Can you work these out from the model? Positions are in its coordinate system, mm. Face numbers are marked on the shaded views. A direction names the side the tool comes from. Coordinates: 2 decimals unless noted, no trailing zeros. Write each loop counter-clockwise with the first axis right and the second up, starting at its lowest first coordinate (ties: lowest second). Pieces come first, ordered by that corner, then holes. Notation, with made-up numbers: (32.25, 33.25) -> (46.25, 33.25) arc R18 cw to (46.25, 46.25) -> close; hole circle Ø3 at (35, 18). An arc over 180 degrees is marked (long way). Use one line per item in the form item = value.
```python
from build123d import *

# Parameters (mm, degrees)
SKETCH1_W           = 60
SKETCH1_H           = 60
BOSS_EXTRUDE1_DEPTH = 6
SKETCH2_W           = 6
SKETCH2_H           = 16
SKETCH2_W_2         = 5.95
SKETCH2_H_2         = 15.95
SKETCH2_W_3         = 5.9
SKETCH2_H_3         = 15.9
SKETCH2_W_4         = 5.85
SKETCH2_H_4         = 15.85
SKETCH2_W_5         = 5.8
SKETCH2_H_5         = 15.8
SKETCH2_W_6         = 5.75
SKETCH2_H_6         = 15.75
CUT_EXTRUDE1_DEPTH  = 6
SKETCH3_W           = 15.128686335
SKETCH3_H           = 1.558081165
CUT_EXTRUDE2_DEPTH  = 6
SKETCH4_W           = 60
SKETCH4_H           = 14.757524832
CUT_EXTRUDE3_DEPTH  = 6


with BuildPart() as part:
    # Sketch1 → Boss-Extrude1 (new body)
    with BuildSketch(Plane(origin=(0, 0, 0), x_dir=(1, 0, 0), z_dir=(0, 1, 0))):
        with Locations((30, 30)):
            Rectangle(SKETCH1_W, SKETCH1_H)
    extrude(amount=BOSS_EXTRUDE1_DEPTH)

    # Sketch2 → Cut-Extrude1 (cut)
    with BuildSketch(Plane(origin=(0, 6, 0), x_dir=(1, 0, 0), z_dir=(0, 1, 0))):
        with Locations((6, 47)):
            Rectangle(SKETCH2_W, SKETCH2_H)
        with Locations((18, 47)):
            Rectangle(SKETCH2_W, SKETCH2_H)
        with Locations((30.15, 47)):
            Rectangle(SKETCH2_W, SKETCH2_H)
        with Locations((42.4, 47)):
            Rectangle(SKETCH2_W, SKETCH2_H)
        with Locations((54.75, 47)):
            Rectangle(SKETCH2_W, SKETCH2_H)
        with Locations((5.975, 25.682524832)):
            Rectangle(SKETCH2_W_2, SKETCH2_H_2)
        with Locations((17.95, 25.707524832)):
            Rectangle(SKETCH2_W_3, SKETCH2_H_3)
        with Locations((30.075, 25.732524832)):
            Rectangle(SKETCH2_W_4, SKETCH2_H_4)
        with Locations((42.3, 25.757524832)):
            Rectangle(SKETCH2_W_5, SKETCH2_H_5)
        with Locations((54.625, 25.782524832)):
            Rectangle(SKETCH2_W_6, SKETCH2_H_6)
    extrude(amount=-CUT_EXTRUDE1_DEPTH, mode=Mode.SUBTRACT)

    # Sketch3 → Cut-Extrude2 (cut)
    with BuildSketch(Plane(origin=(0, 6, 0), x_dir=(1, 0, 0), z_dir=(0, 1, 0))):
        with Locations((30.785905784, 59.220959418)):
            Rectangle(SKETCH3_W, SKETCH3_H)
    extrude(amount=-CUT_EXTRUDE2_DEPTH, mode=Mode.SUBTRACT)

    # Sketch4 → Cut-Extrude3 (cut)
    with BuildSketch(Plane(origin=(0, 6, 0), x_dir=(1, 0, 0), z_dir=(0, 1, 0))):
        with Locations((30, 7.378762416)):
            Rectangle(SKETCH4_W, SKETCH4_H)
    extrude(amount=-CUT_EXTRUDE3_DEPTH, mode=Mode.SUBTRACT)


solid = part.part
```
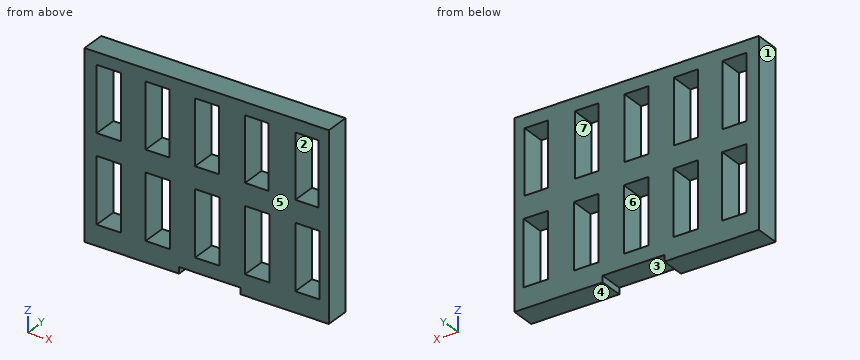
Q1. Suppose I cut it at D-D (y = 3.4). Give the number of separate pieces and of enclosed holes in the cut face, then the cut area to 3 significant figures.
Return value:
separate_pieces = 1
enclosed_holes = 10
area = 1,750 mm2
Q2. If I drill on line 1 (X direction, y = 3.75, z = -43.5); line 2 (Z direction, x = 56, y = 5.45); line 3 (X direction, y = 4, z = -18), over which ranges is the centre line in solid material (lowest first)? Write a range as from..to.
Return value:
line_1 = 0..3, 9..15, 21..27.15, 33.15..39.4, 45.4..51.75, 57.75..60
line_2 = -60..-55, -39..-33.66, -17.91..-14.76
line_3 = 0..3, 8.95..15, 20.9..27.15, 33..39.4, 45.2..51.75, 57.5..60
Q3. Thinking about a two-plate mould opening in Z: for the marked faces 4, 5, 6 and 7, which applies, released by +Z, released by -Z, zero draft, split by the parting line, or undercut?
Return value:
face_4 = released by -Z
face_5 = zero draft
face_6 = undercut
face_7 = undercut
Q4. Suppose I cut it at C-C (x = 8). Write out the boundary of the cut face in (y, z), then the cut area to 3 significant figures.
Return value:
outline = (0, -60) -> (6, -60) -> (6, -55) -> (0, -55) -> close; (0, -39) -> (6, -39) -> (6, -33.66) -> (0, -33.66) -> close; (0, -17.71) -> (6, -17.71) -> (6, -14.76) -> (0, -14.76) -> close
area = 79.8 mm2
Q5. Suppose I cut it at B-B (z = -47). Write out the boundary of the cut face in (x, y), then the cut area to 3 significant figures.
Return value:
outline = (0, 0) -> (3, 0) -> (3, 6) -> (0, 6) -> close; (9, 0) -> (15, 0) -> (15, 6) -> (9, 6) -> close; (21, 0) -> (27.15, 0) -> (27.15, 6) -> (21, 6) -> close; (33.15, 0) -> (39.4, 0) -> (39.4, 6) -> (33.15, 6) -> close; (45.4, 0) -> (51.75, 0) -> (51.75, 6) -> (45.4, 6) -> close; (57.75, 0) -> (60, 0) -> (60, 6) -> (57.75, 6) -> close
area = 180 mm2
Q6. Suppose I cut it at A-A (x = 53). Write out the boundary of the cut face in (y, z), then the cut area to 3 significant figures.
Return value:
outline = (0, -60) -> (6, -60) -> (6, -55) -> (0, -55) -> close; (0, -39) -> (6, -39) -> (6, -33.66) -> (0, -33.66) -> close; (0, -17.91) -> (6, -17.91) -> (6, -14.76) -> (0, -14.76) -> close
area = 81.0 mm2
Q7. For the marked faces 1, 2 and 3, which set-ups out of +Z, -Z, +X, -X, +Y, -Y let a thin tool reach every point of the face, with its end or its side?
Return value:
face_1 = +Z, -Z, -X, +Y, -Y
face_2 = +Y, -Y
face_3 = -Z, +Y, -Y
Q8. Will this pin go through, and if not, where does the flat tip stop? pin 1 (3 mm diameter, centred on x = 29, y = 4, fed in from -Z).
Return value:
pin_1 = -58.44
